Here's how the part is built. I have some questions about the finished solid (model axes, mm). A direction names the side the tool comes from. Round coordinates to 2 decimals unless told otherwise and drop trailing zeros. Write each loop counter-clockwise with the first axis right and the second up, starting at its lowest first coordinate (ties: lowest second). Pieces come first, ordered by that corner, then holes. Notation, with made-up numbers: (64, -38.75) -> (93, -38.75) arc R15 cw to (93, -25.75) -> close; hole circle Ø6 at (32, -35). An arc over 180 degrees is marked (long way). Answer in a Markdown table with one row per item.
from build123d import *

# Parameters (mm, degrees)
SKETCH2_R               = 9
BOSS_EXTRUDE1_DEPTH     = 10
SKETCH3_R               = 6
CUT_EXTRUDE1_DEPTH      = 53
CHAMFER1_SIZE           = 4
FILLET4_R               = 1
SKETCH8_W               = 10
SKETCH8_H               = 21.176663605
CUT_EXTRUDE3_DEPTH      = 31
CUT_EXTRUDE3_DEPTH_BACK = 31
SKETCH10_R              = 13.1
CUT_EXTRUDE4_DEPTH      = 10


with BuildPart() as part:
    # Sketch1 → Revolve1 (revolve)
    with BuildSketch(Plane.XY):
        Polygon((-21, 0), (21, 0), (21, 30), (9, 30), (9, 15), (-9, 15), (-9, 30), (-21, 30), align=None)
    revolve(axis=Axis((-21, 0, 0), (1, 0, 0)))

    # Sketch2 → Boss-Extrude1 (add)
    with BuildSketch(Plane(origin=(21, 0, 0), x_dir=(0, 0, -1), z_dir=(1, 0, 0))):
        Circle(SKETCH2_R)
    extrude(amount=BOSS_EXTRUDE1_DEPTH)

    # Sketch3 → Cut-Extrude1 (cut, through all)
    with BuildSketch(Plane(origin=(31, 0, 0), x_dir=(0, 0, -1), z_dir=(1, 0, 0))):
        Circle(SKETCH3_R)
    extrude(amount=-CUT_EXTRUDE1_DEPTH, mode=Mode.SUBTRACT)

    # Chamfer1
    chamfer1_edges = [part.edges().sort_by_distance(p)[0] for p in [
        (-9, -30, 0),
        (9, -30, 0),
    ]]
    chamfer(chamfer1_edges, length=CHAMFER1_SIZE)

    # Fillet4
    fillet4_edges = [part.edges().sort_by_distance(p)[0] for p in [
        (-21, -30, 0),
        (21, -30, 0),
    ]]
    fillet(fillet4_edges, radius=FILLET4_R)

    # Sketch8 → Cut-Extrude3 (cut, two sides)
    with BuildSketch(Plane(origin=(0, 0, 0), x_dir=(1, 0, 0), z_dir=(0, 1, 0))) as cut_extrude3_sk:
        with Locations((26, 0.476968454)):
            Rectangle(SKETCH8_W, SKETCH8_H)
    extrude(amount=CUT_EXTRUDE3_DEPTH, mode=Mode.SUBTRACT)
    extrude(cut_extrude3_sk.sketch, amount=-CUT_EXTRUDE3_DEPTH_BACK, mode=Mode.SUBTRACT)

    # Sketch10 → Cut-Extrude4 (cut)
    with BuildSketch(Plane(origin=(21, 0, 0), x_dir=(0, 0, -1), z_dir=(1, 0, 0))):
        Circle(SKETCH10_R)
    extrude(amount=-CUT_EXTRUDE4_DEPTH, mode=Mode.SUBTRACT)


solid = part.part
1) We'd pull the mould along Y, two halves only. Please class faces 4 (the face through (11, -3, -6)), 5 (the face through (16.45, -29.97, 1.32)), 6 (the face through (-21, 0, 7)): +Y half, -Y half, draft (parallel to the pull), parting line (faces both ways), or undercut.
Response:
| item | result |
|---|---|
| face 4 | undercut |
| face 5 | parting line |
| face 6 | draft |
2) Which directions (+Z, -Z, +X, -X, +Y, -Y) give clear straight access to the entire face, cutting with the end or side of a thin tool? Please do faces 1 (the face through (16.07, 12.989, 1.705)), 2 (the face through (-16.55, -29.97, 1.32)), 3 (the face through (9, 11, -11)).
Response:
| item | result |
|---|---|
| face 1 | +X |
| face 2 | +X, -X |
| face 3 | none |
3) I want a section at A-A, the plane z = 0. List the corners of the cut face in (x, y) for me.
Response:
| item | result |
|---|---|
| outline | (-21, -29) arc R1 ccw to (-20, -30) -> (-13, -30) -> (-9, -26) -> (-9, -15) -> (9, -15) -> (9, -26) -> (13, -30) -> (20, -30) arc R1 ccw to (21, -29) -> (21, -13.1) -> (11, -13.1) -> (11, -6) -> (-21, -6) -> close; (-21, 6) -> (11, 6) -> (11, 13.1) -> (21, 13.1) -> (21, 29) arc R1 ccw to (20, 30) -> (13, 30) -> (9, 26) -> (9, 15) -> (-9, 15) -> (-9, 26) -> (-13, 30) -> (-20, 30) arc R1 ccw to (-21, 29) -> close |
4) I want a section at C-C, the plane x = -15. List the corners of the cut face in (y, z) for me.
Response:
| item | result |
|---|---|
| outline | circle Ø60 at (0, 0); hole circle Ø12 at (0, 0) |
5) I need wall thicknesses on line 1 (X direction, y = 5, z = -17.5); line 2 (Y direction, x = -12, z = -1); line 3 (X direction, y = 9, z = -8). Which ranges of each line are inside material? Lowest first, please. Write a range as [from, to].
Response:
| item | result |
|---|---|
| line 1 | x = [-21, -9], [9, 21] |
| line 2 | y = [-28.98, -5.92], [5.92, 28.98] |
| line 3 | x = [-21, 11] |
6) For pin 1 (12 mm diameter, centred on x = -0.5, y = -15, fed in from +Z); pin 2 (8 mm diameter, centred on y = -2.5, z = -3.5, fed in from +X); pin 3 (3 mm diameter, centred on x = 14, z = -23, fed in from -Y), each with a flat end and sliding along its axis, tell me the tip position at first contact or that it passes through.
Response:
| item | result |
|---|---|
| pin 1 | stops at z = 12 |
| pin 2 | stops at x = 11 |
| pin 3 | stops at y = -20.92 |
7) I want a section at D-D, the plane x = 12. List the corners of the cut face in (y, z) for me.
Response:
| item | result |
|---|---|
| outline | circle Ø58 at (0, 0); hole circle Ø26.2 at (0, 0) |
